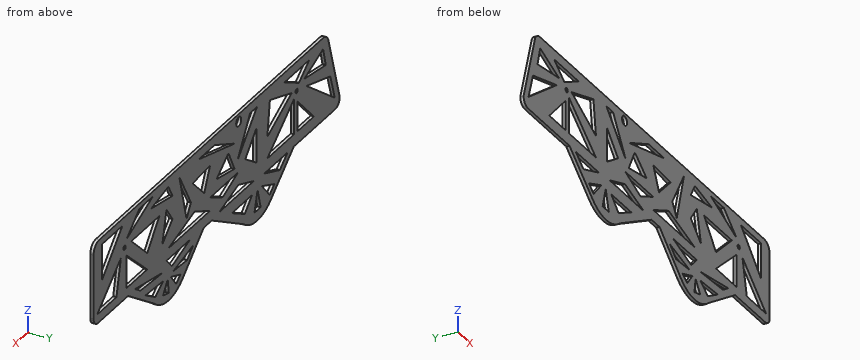
```python
from build123d import *

# Parameters (mm, degrees)
SKETCH1_R           = 2
SKETCH1_R_2         = 4.313560469
SKETCH1_R_3         = 4.5
SKETCH1_R_4         = 3.716178426
BOSS_EXTRUDE1_DEPTH = 3.175
SKETCH2_W           = 597.466303312
SKETCH2_H           = 60.972543052
CUT_EXTRUDE1_DEPTH  = 70
FILLET1_R           = 10
FILLET2_R           = 10
SKETCH6_R           = 40
BOSS_EXTRUDE2_DEPTH = 3.175
BOSS_EXTRUDE3_DEPTH = 3.175
SKETCH9_R           = 40
BOSS_EXTRUDE4_DEPTH = 3.175
BOSS_EXTRUDE6_DEPTH = 3.175
CUT_EXTRUDE2_DEPTH  = 10
CUT_EXTRUDE3_DEPTH  = 10
CUT_EXTRUDE4_DEPTH  = 10
CUT_EXTRUDE5_DEPTH  = 10
CUT_EXTRUDE6_DEPTH  = 10


with BuildPart() as part:
    # Sketch1 → Boss-Extrude1 (new body)
    with BuildSketch(Plane(origin=(0, 0, 0), x_dir=(1, 0, 0), z_dir=(0, 1, 0))):
        with BuildLine():
            ThreePointArc((8, 150), (2.343145751, 147.656854249), (0, 142))
            Line((0, 142), (42, 8))
            ThreePointArc((42, 8), (44.343145751, 2.343145751), (50, 0))
            Line((50, 0), (436.5, 0))
            ThreePointArc((436.5, 0), (442.156854249, 2.343145751), (444.5, 8))
            Line((444.5, 8), (444.5, 142))
            ThreePointArc((444.5, 142), (442.156854249, 147.656854249), (436.5, 150))
            Line((436.5, 150), (336.748623665, 150))
            ThreePointArc((336.748623665, 150), (334.106475607, 148.038018595), (331.46432755, 150))
            Line((331.46432755, 150), (8, 150))
        make_face()
        with Locations(Location((388.475756445, 100.077126905, 0), (0, 0, 270))):
            Circle(SKETCH1_R, mode=Mode.SUBTRACT)
        with Locations(Location((307.606475607, 140.710564477, 0), (0, 0, 270))):
            Circle(SKETCH1_R_2, mode=Mode.SUBTRACT)
        with Locations(Location((77.821750814, 98.327219393, 0), (0, 0, 270))):
            Circle(SKETCH1_R, mode=Mode.SUBTRACT)
        with Locations(Location((182.429479385, 77.355745695, 0), (0, 0, 270))):
            Circle(SKETCH1_R_3, mode=Mode.SUBTRACT)
        with Locations(Location((146.269370224, 139.84039861, 0), (0, 0, 270))):
            Circle(SKETCH1_R_4, mode=Mode.SUBTRACT)
    extrude(amount=BOSS_EXTRUDE1_DEPTH)

    # Sketch2 → Cut-Extrude1 (cut)
    with BuildSketch(Plane.XY):
        with Locations((220.1785332, 7.544358636)):
            Rectangle(SKETCH2_W, SKETCH2_H)
    extrude(amount=-CUT_EXTRUDE1_DEPTH, mode=Mode.SUBTRACT)

    # Fillet1
    fillet1_edges = [part.edges().sort_by_distance(p)[0] for p in [
        (22.567164179, 1.5875, -70),
    ]]
    fillet(fillet1_edges, radius=FILLET1_R)

    # Fillet2
    fillet2_edges = [part.edges().sort_by_distance(p)[0] for p in [
        (444.5, 1.5875, -70),
    ]]
    fillet(fillet2_edges, radius=FILLET2_R)

    # Sketch6 → Boss-Extrude2 (add)
    with BuildSketch(Plane(origin=(0, 0, 0), x_dir=(1, 0, 0), z_dir=(0, 1, 0))):
        with Locations((149, 150.04039861)):
            Circle(SKETCH6_R)
    extrude(amount=BOSS_EXTRUDE2_DEPTH)

    # Sketch7 → Boss-Extrude3 (add)
    with BuildSketch(Plane(origin=(0, 0, 0), x_dir=(1, 0, 0), z_dir=(0, 1, 0))):
        Polygon((124.164543783, 181.396420591), (82.702881078, 149.750534228), (231.468946681, 149.750534228), (173.835456217, 181.396420591), align=None)
    extrude(amount=BOSS_EXTRUDE3_DEPTH)

    # Sketch9 → Boss-Extrude4 (add)
    with BuildSketch(Plane(origin=(0, 0, 0), x_dir=(1, 0, 0), z_dir=(0, 1, 0))):
        with BuildLine():
            ThreePointArc((269, 150), (272.870833001, 167.166341835), (283.734164599, 181.010281545))
            Line((283.734164599, 181.010281545), (245.673378314, 150))
            Line((245.673378314, 150), (269, 150))
        make_face()
        with Locations((309, 150)):
            Circle(SKETCH9_R)
    extrude(amount=BOSS_EXTRUDE4_DEPTH)

    # Sketch12 → Boss-Extrude6 (add)
    with BuildSketch(Plane(origin=(0, 0, 0), x_dir=(1, 0, 0), z_dir=(0, 1, 0))):
        Polygon((326.166341835, 186.129166999), (382.106475607, 150), (340.398839744, 150), align=None)
    extrude(amount=BOSS_EXTRUDE6_DEPTH)

    # Sketch13 → Cut-Extrude2 (cut)
    with BuildSketch(Plane(origin=(0, 3.175, 0), x_dir=(1, 0, 0), z_dir=(0, 1, 0))):
        Polygon((126.596630185, 175.699600472), (118.071388699, 169.473803102), (140.590780828, 160.520909874), align=None)
        Polygon((142.805778665, 179.955358976), (153.92453015, 179.955358976), (148.365154407, 160.520909874), align=None)
        Polygon((158.369799386, 160.520909874), (171.45690463, 172.586701787), (194.594159282, 160.520909874), align=None)
        Polygon((108.223756098, 160.520909874), (94.177153866, 150.262983529), (136.512601507, 150.262983529), align=None)
        Polygon((155.324532982, 148.431005589), (192.465847063, 148.431005589), (217.292214981, 148.431005589), (183.025531956, 138.62875365), align=None)
    extrude(amount=-CUT_EXTRUDE2_DEPTH, mode=Mode.SUBTRACT)

    # Sketch14 → Cut-Extrude3 (cut)
    with BuildSketch(Plane(origin=(0, 3.175, 0), x_dir=(1, 0, 0), z_dir=(0, 1, 0))):
        Polygon((287.387365491, 175.190284075), (295.66806948, 180.292754759), (305.015851869, 168.900328202), align=None)
        Polygon((308.630084677, 182.834690248), (318.900148429, 180.292754759), (310.630809682, 168.900328202), align=None)
        Polygon((318.900148429, 166.379196716), (332.89720101, 175.004012981), (350.750845105, 164.702889414), align=None)
        Polygon((300.341960675, 165.541043065), (275.583975015, 166.844059842), (264.607664644, 157.837711611), align=None)
        Polygon((318.900148429, 157.837711611), (359.859445758, 155.682017188), (369.45606502, 149.484000906), align=None)
        Polygon((302.829713803, 159.399721535), (270.095819829, 149.484000906), (312.697737902, 149.484000906), align=None)
    extrude(amount=-CUT_EXTRUDE3_DEPTH, mode=Mode.SUBTRACT)

    # Sketch15 → Cut-Extrude4 (cut)
    with BuildSketch(Plane(origin=(0, 3.175, 0), x_dir=(1, 0, 0), z_dir=(0, 1, 0))):
        Polygon((9.082536395, 138.332869462), (16.951784082, 113.666673792), (59.847245845, 102.198186546), align=None)
        Polygon((46.527345648, 138.332869462), (75.932780446, 138.332869462), (75.932780446, 109.552219535), align=None)
        Polygon((82.275228769, 103.765733182), (130.726352108, 138.332869462), (82.275228769, 138.332869462), align=None)
        Polygon((25.252080853, 98.620149784), (30.014206453, 80.800449194), (63.923719137, 93.326510285), align=None)
        Polygon((73.651734719, 92.462114854), (55.153094423, 79.264381219), (99.755557686, 79.264381219), align=None)
        Polygon((86.703646203, 95.973330035), (130.726352108, 117.260863799), (126.131589339, 83.694731493), align=None)
    extrude(amount=-CUT_EXTRUDE4_DEPTH, mode=Mode.SUBTRACT)

    # Sketch16 → Cut-Extrude5 (cut)
    with BuildSketch(Plane(origin=(0, 3.175, 0), x_dir=(1, 0, 0), z_dir=(0, 1, 0))):
        Polygon((437.892195527, 140.994591207), (395.306902067, 107.113261781), (403.121369003, 140.994591207), align=None)
        Polygon((384.654839472, 93.268223937), (361.655164528, 74.969428739), (337.798732838, 74.969428739), align=None)
        Polygon((429.106942721, 111.483374831), (392.46021732, 76.762265555), (429.106942721, 76.762265555), align=None)
        Polygon((384.654839472, 140.994591207), (347.551515413, 140.994591207), (384.654839472, 109.39285335), align=None)
        Polygon((347.551515413, 125.193722279), (325.746359439, 99.592479337), (376.307639908, 99.592479337), align=None)
    extrude(amount=-CUT_EXTRUDE5_DEPTH, mode=Mode.SUBTRACT)

    # Sketch17 → Cut-Extrude6 (cut)
    with BuildSketch(Plane(origin=(0, 3.175, 0), x_dir=(1, 0, 0), z_dir=(0, 1, 0))):
        Polygon((234.14639503, 139.026116815), (309.197820801, 139.026116815), (262.118798526, 126.26771918), align=None)
        Polygon((211.155668978, 136.962371774), (183.727319265, 126.26771918), (234.14639503, 126.26771918), align=None)
        Polygon((150.710604994, 132.646917997), (150.710604994, 99.742633834), (170.588020135, 119.620048974), align=None)
        Polygon((150.710604994, 80.176001915), (184.553616381, 114.019013303), (161.611869132, 79.012701862), (149.369026486, 79.012701862), align=None)
        Polygon((190.022281375, 95.03260673), (225.996651018, 79.012701862), (254.545180422, 79.012701862), align=None)
        Polygon((200.527414873, 99.742633834), (190.022281375, 119.620048974), (222.283730898, 114.019013303), (202.008756576, 99.742633834), align=None)
        Polygon((244.72715064, 116.819531138), (234.14639503, 95.03260673), (265.507593925, 97.097507609), align=None)
        Polygon((268.717573549, 114.019013303), (289.655742431, 79.012701862), (276.569858899, 126.26771918), align=None)
        Polygon((301.929754413, 114.019013303), (320.262459356, 129.915538559), (312.771055987, 99.742633834), align=None)
        Polygon((301.929754413, 91.509886863), (309.404639922, 79.012701862), (340.535394318, 85.261294363), align=None)
    extrude(amount=-CUT_EXTRUDE6_DEPTH, mode=Mode.SUBTRACT)


solid = part.part
```
Source: CAD feature listing. Evaluate the final solid. Frame: model axes, mm. Give positions to 0.01 mm unless a question says otherwise; leave off trailing zeros. Order: outer loops, then holes, each group sorted by start corner. A loop starts at its lowest first (then second) coordinate and runs counter-clockwise, first axis right, second up.
(1) Material intervals for line 1 along Z through (x, y) = (100, 1.8); line 2 along Z through (x, y) = (293, 2.15); line 3 along Z through (x, y) = (293.5, 2.1), sorted ascending.
(2) Section query B-B (y = 0.65). State how many separate pieces and enclosed holes the cut face has, plus the area to 3 significant figures.
(3) Section query A-A (x = 417). Return the cut outline in (y, z) (3 decimals).
(4) Contact query for flat-ended pins moving along their axis: P1, Ø1, axis at x = 199, y = 2.5, coming from the -Z side; P2, Ø1.6, axis at x = 292.5, y = 1, coming from the -Z side; P3, Ø1, axis at x = 73, y = 1, coming from the -Z side. Output: stop coordinate, or through.
Outcome:
1. line 1: z = -162.95 to -154.52, -150.26 to -138.33, -116.41 to -102.4, -91.83 to -70
1. line 2: z = -186.66 to -178.65, -173.19 to -165.93, -163.96 to -156.42, -149.48 to -139.03, -134.64 to -70
1. line 3: z = -186.87 to -178.96, -173.01 to -165.9, -164.07 to -156.57, -149.48 to -139.03, -134.77 to -70
2. separate pieces: 1
2. enclosed holes: 35
2. area: 30,900 mm2
3. outline: (0, -150) - (3.175, -150) - (3.175, -140.995) - (0, -140.995) - close; (0, -124.373) - (3.175, -124.373) - (3.175, -100.013) - (0, -100.013) - close; (0, -76.762) - (3.175, -76.762) - (3.175, -70) - (0, -70) - close
4. P1: stops at z = -167.85
4. P2: stops at z = -186.79
4. P3: stops at z = -150
